Autodesk Inventor part; units mm, degrees
ref_plane "YZ Plane" through (0, 0, 0) normal (1, 0, 0) x (0, 1, 0)
ref_plane "XZ Plane" through (0, 0, 0) normal (0, 1, 0) x (-1, 0, 0)
ref_plane "XY Plane" through (0, 0, 0) normal (0, 0, 1) x (1, 0, 0)
sketch "Sketch1" plane through (0, 0, 0) normal (1, 0, 0) x (0, 1, 0)
  line L0 (0, 0) -> (0, 0)
  line L1 (25.4, 0) -> (25.4, 12.7)
  line L2 (12.7, 25.4) -> (0, 25.4)
  line L3 (0, 25.4) -> (0, 0)
  line L4 (12.7, -238.6076) -> (0, -238.6076)
  line L5 (0, -238.6076) -> (0, -213.2076)
  line L6 (0, -213.2076) -> (0, -213.2076)
  line L7 (25.4, -213.2076) -> (25.4, -225.9076)
  arc A0 (25.4, 12.7) -> (12.7, 25.4) centre (12.7, 12.7) ccw
  arc A1 (12.7, -238.6076) -> (25.4, -225.9076) centre (12.7, -225.9076) ccw
  arc A2 (6.35, -12.7) -> (0, 0) centre (-8.8867, -12.3808) ccw
  arc A3 (0, -213.2076) -> (6.35, -200.5076) centre (-8.8867, -200.8268) ccw
  line L8 (25.4, 0) -> (25.4, -213.2076)
  line L9 (6.35, -200.5076) -> (6.35, -12.7)
  point P0 (0, -213.2076)
  point P1 (0, -213.2076)
  dimension "d5" = 25.4
  dimension "d6" = 12.7
  dimension "d9" = 264.0076
  dimension "d10" = 25.4
  dimension "d12" = 25.4
  dimension "d15" = 15.24
  dimension "d16" = 15.24
extrude "Extrusion1" add sketch "Sketch1" along normal mid plane 19.05
sketch "Sketch2" plane through (-9.525, 0, 0) normal (0, -1, 0) x (1, 0, 0)
  line L0 (0, 0) -> (19.05, 0)
  line L1 (19.05, 12.7) -> (19.05, 25.4)
  line L2 (0, 0) -> (19.05, 0)
  line L3 (19.05, 0) -> (19.05, 25.4)
  line L4 (19.05, 25.4) -> (0, 25.4)
  line L5 (0, 25.4) -> (0, 0)
  line L6 (0, -213.2076) -> (19.05, -213.2076)
  line L7 (0, -238.6076) -> (19.05, -238.6076)
  line L8 (19.05, -213.2076) -> (0, -213.2076)
  line L9 (0, -213.2076) -> (0, -238.6076)
  line L10 (0, -238.6076) -> (19.05, -238.6076)
  line L11 (19.05, -238.6076) -> (19.05, -213.2076)
  line L12 (25.4, -206.8576) -> (-6.35, -206.8576)
  line L13 (-6.35, -206.8576) -> (-6.35, -244.9576)
  line L14 (25.4, -244.9576) -> (25.4, -206.8576)
  line L15 (-6.35, -6.35) -> (25.4, -6.35)
  line L16 (25.4, -6.35) -> (25.4, 31.75)
  line L17 (-6.35, 31.75) -> (-6.35, -6.35)
  line L18 (-6.35, 44.45) -> (25.4, 44.45)
  line L19 (25.4, 44.45) -> (25.4, 31.75)
  line L20 (-6.35, 31.75) -> (-6.35, 44.45)
  line L21 (-6.35, -244.9576) -> (-6.35, -257.6576)
  line L22 (-6.35, -257.6576) -> (25.4, -257.6576)
  line L23 (25.4, -257.6576) -> (25.4, -244.9576)
  point P0 (9.525, 0)
  dimension "d17" = 31.75
  dimension "d18" = 38.1
  dimension "d19" = 31.75
  dimension "d20" = 38.1
  dimension "d23" = 12.7
extrude "Extrusion2" add sketch "Sketch2" against normal blind 6.35 contours L5 L4 L1 L3 L0 | L6 L11 L7 L9 | L14 L23 L22 L21 L13 L12 | L17 L20 L18 L19 L16 L15
sketch "Sketch3" plane through (-9.525, 6.35, 0) normal (0, 1, 0) x (1, 0, 0)
  circle A0 centre (0, 251.3076) radius 2.54
  circle A1 centre (19.05, 251.3076) radius 2.54
  line L0 (25.4, 206.8576) -> (25.4, 257.6576)
  line L1 (25.4, 257.6576) -> (-6.35, 257.6576)
  line L2 (-6.35, 257.6576) -> (-6.35, 206.8576)
  circle A2 centre (0, -38.1) radius 2.54
  circle A3 centre (19.05, -38.1) radius 2.54
  line L3 (-6.35, 6.35) -> (-6.35, -44.45)
  line L4 (-6.35, -44.45) -> (25.4, -44.45)
  line L5 (25.4, -44.45) -> (25.4, 6.35)
  point P0 (9.525, 0)
  dimension "d24" = 5.08
  dimension "d25" = 5.08
  dimension "d26" = 6.35
  dimension "d27" = 6.35
  dimension "d28" = 6.35
  dimension "d29" = 6.35
  dimension "d30" = 5.08
  dimension "d31" = 5.08
  dimension "d32" = 6.35
  dimension "d33" = 6.35
  dimension "d34" = 6.35
  dimension "d35" = 6.35
extrude "Extrusion3" cut sketch "Sketch3" against normal through all
sketch "Sketch4" plane through (9.525, 0, 0) normal (1, 0, 0) x (0, 0, -1)
  line L0 (200.5076, 6.35) -> (12.7, 6.35)
  line L1 (87.5538, 0) -> (125.6538, 0)
  line L2 (125.6538, 0) -> (125.6538, 6.35)
  line L3 (125.6538, 6.35) -> (87.5538, 6.35)
  line L4 (87.5538, 6.35) -> (87.5538, 0)
  line L5 (87.5538, 0) -> (125.6538, 6.35) construction
  line L6 (125.6538, 0) -> (87.5538, 6.35) construction
  point P0 (0, 0)
  point P1 (106.6038, 6.35)
  point P2 (106.6038, 3.175)
  dimension "d38" = 38.1
extrude "Extrusion4" add sketch "Sketch4" against normal blind 19.05
fillet "Fillet1" radius 1.5875 14 edges at (15.875, 6.35, 19.05) (0, 6.35, 25.4) (9.525, 6.35, 9.525) (0, 6.35, 44.45) (-15.875, 6.35, 19.05) (-9.525, 6.35, 9.525) (0, 0, -125.6538) (0, 0, -87.5538) (9.525, 6.35, -222.7326) (15.875, 6.35, -232.2576) (0, 6.35, -238.6076) (0, 6.35, -257.6576) (-9.525, 6.35, -222.7326) (-15.875, 6.35, -232.2576)
properties part number "IndexRailM" material "Polycarbonate, Clear"
CAD build for the part. Positions are in the model's coordinates, mm. A direction names the side the tool comes from. Round coordinates to 2 decimals unless told otherwise and drop trailing zeros. Order: outer loops, then holes, each group sorted by start corner. A loop starts at its lowest first (then second) coordinate and runs counter-clockwise, first axis right, second up.
Item 1: Tool access for faces 1 (the face through (0, 4, -125.654)), 2 (the face through (0, 10, -238.608)), 3 (the face through (0, 10, 25.4)): list every direction of +Z, -Z, +X, -X, +Y, -Y with a clear straight run to the whole face (end or side of a thin tool).
Item 2: Mould opens along X. For faces 4 (the face through (-10.08, 3.22, 40.58)), 5 (the face through (0, 6.35, -164)), 6 (the face through (15.875, 2, 19)) say: pulls with the +X half, pulls with the -X half, needs draft (parallel to the pull), parting line crosses it, or undercut.
Item 3: Saw through at A-A on z = 38.1. State how many separate pieces and enclosed holes the cut face has, then the cut area to 3 significant figures.
Item 4: Pin check, flat tips, straight feed: pin 1 (8.5 mm diameter, centred on x = -3, z = -234.5, fed in from +Y); pin 2 (2.5 mm diameter, centred on x = -1.5, y = 10, fed in from -Z); pin 3 (2 mm diameter, centred on x = -2.5, y = 12.5, fed in from +Z); pin 4 (3 mm diameter, centred on x = 9.525, z = 38.1, fed in from -Y). Stop position of each tip, or through.
Item 5: Saw through at C-C on z = -34. Write the cut outline in (x, y) (3 decimals).
Item 6: Probe line 1 along Z through (x, y) = (2, 2.5); line 2 along Y through (x, z) = (4, -34.5); line 3 along Y through (x, z) = (-1, -89). List the from-to ranges inside material, lowest first.
Reported:
1. face 1: +X, -X, -Y
1. face 2: -Z, +X, -X, +Y
1. face 3: +Z, +X, -X, +Y
2. face 4: undercut
2. face 5: needs draft
2. face 6: pulls with the +X half
3. separate pieces: 3
3. enclosed holes: 0
3. area: 136 mm2
4. pin 1: stops at y = 24.63
4. pin 2: stops at z = -238.61
4. pin 3: stops at z = 25.4
4. pin 4: passes through
5. outline: (-9.525, 6.35) - (9.525, 6.35) - (9.525, 25.4) - (-9.525, 25.4) - close
6. line 1: z = -257.66 to -206.86, -125.65 to -87.55, -6.35 to 44.45
6. line 2: y = 6.35 to 25.4
6. line 3: y = 0.01 to 25.4
